Source: CAD feature listing. Evaluate the final solid. Frame: model axes, mm. Face numbers are marked on the shaded views. A direction names the side the tool comes from. Give positions to 0.01 mm unless a question says otherwise; leave off trailing zeros. Loops run counter-clockwise (first coordinate to the right, second up) from the corner with the lowest first, then second, coordinate; pieces in that order, holes last.
from build123d import *

# Parameters (mm, degrees)
F0_R     = 11.176
F0_R_2   = 6.35
F1_DEPTH = 19.05
F2_DEPTH = 6.35
F3_DEPTH = 31.75
F5_DEPTH = 19.05
F6_DEPTH = 50.8


with BuildPart() as f1:
    # F0 (on Top) → F1 (new body)
    with BuildSketch(Plane.XY):
        with BuildLine():
            ThreePointArc((-44.45, 25.4), (-69.85, 0), (-44.45, -25.4))
            Line((-44.45, -25.4), (2.63e-08, -25.4))
            ThreePointArc((2.63e-08, -25.4), (-25.4, -1.24e-08), (1.5e-09, 25.4))
            Line((1.5e-09, 25.4), (-44.45, 25.4))
        make_face()
        with Locations((-44.45, 0)):
            Circle(F0_R, mode=Mode.SUBTRACT)
        with BuildLine():
            ThreePointArc((25.4, 0), (17.9605122514, -17.9605122328), (2.63e-08, -25.4))
            Line((2.63e-08, -25.4), (44.45, -25.4))
            ThreePointArc((44.45, -25.4), (69.85, 0), (44.45, 25.4))
            Line((44.45, 25.4), (1.5e-09, 25.4))
            ThreePointArc((1.5e-09, 25.4), (17.9605122427, 17.9605122416), (25.4, 0))
        make_face()
        with Locations((44.45, 0)):
            Circle(F0_R, mode=Mode.SUBTRACT)
        with Locations((-44.45, 0)):
            Circle(F0_R)
        with Locations((-44.45, 0)):
            Circle(F0_R_2, mode=Mode.SUBTRACT)
        with Locations((44.45, 0)):
            Circle(F0_R)
        with Locations((44.45, 0)):
            Circle(F0_R_2, mode=Mode.SUBTRACT)
        with BuildLine():
            ThreePointArc((1.5e-09, 25.4), (-25.4, -1.24e-08), (2.63e-08, -25.4))
            ThreePointArc((2.63e-08, -25.4), (17.9605122514, -17.9605122328), (25.4, 0))
            ThreePointArc((25.4, 0), (17.9605122427, 17.9605122416), (1.5e-09, 25.4))
        make_face()
    extrude(amount=-F1_DEPTH)

    # F0 (on Top) → F2 (cut)
    with BuildSketch(Plane.XY):
        with Locations((-44.45, 0)):
            Circle(F0_R)
        with Locations((-44.45, 0)):
            Circle(F0_R_2, mode=Mode.SUBTRACT)
        with Locations((44.45, 0)):
            Circle(F0_R)
        with Locations((44.45, 0)):
            Circle(F0_R_2, mode=Mode.SUBTRACT)
    extrude(amount=-F2_DEPTH, mode=Mode.SUBTRACT)

    # F0 (on Top) → F3 (join)
    with BuildSketch(Plane.XY):
        with BuildLine():
            ThreePointArc((1.5e-09, 25.4), (-25.4, -1.24e-08), (2.63e-08, -25.4))
            ThreePointArc((2.63e-08, -25.4), (17.9605122514, -17.9605122328), (25.4, 0))
            ThreePointArc((25.4, 0), (17.9605122427, 17.9605122416), (1.5e-09, 25.4))
        make_face()
    extrude(amount=F3_DEPTH)

    # F4 (on face) → F5 (cut)
    with BuildSketch(Plane.XY.offset(31.75)):
        with BuildLine():
            Line((6.35, -24.5934442484), (6.35, -12.8696814646))
            ThreePointArc((6.35, -12.8696814646), (0, -14.351), (-6.35, -12.8696814646))
            Line((-6.35, -12.8696814646), (-6.35, -24.5934442484))
            ThreePointArc((-6.35, -24.5934442484), (0, -25.4), (6.35, -24.5934442484))
        make_face()
        with BuildLine():
            ThreePointArc((-12.8696814646, -6.35), (-14.351, 0), (-12.8696814646, 6.35))
            Line((-12.8696814646, 6.35), (-24.5934442484, 6.35))
            ThreePointArc((-24.5934442484, 6.35), (-25.4, 0), (-24.5934442484, -6.35))
            Line((-24.5934442484, -6.35), (-12.8696814646, -6.35))
        make_face()
        with BuildLine():
            ThreePointArc((-6.35, 12.8696814646), (0, 14.351), (6.35, 12.8696814646))
            Line((6.35, 12.8696814646), (6.35, 24.5934442484))
            ThreePointArc((6.35, 24.5934442484), (0, 25.4), (-6.35, 24.5934442484))
            Line((-6.35, 24.5934442484), (-6.35, 12.8696814646))
        make_face()
        with BuildLine():
            ThreePointArc((12.8696814646, 6.35), (13.9757647322, 3.260245566), (14.351, 0))
            ThreePointArc((14.351, 0), (13.9757647322, -3.260245566), (12.8696814646, -6.35))
            Line((12.8696814646, -6.35), (24.5934442484, -6.35))
            ThreePointArc((24.5934442484, -6.35), (25.1975542852, -3.2005090291), (25.4, 0))
            ThreePointArc((25.4, 0), (25.1975542852, 3.2005090291), (24.5934442484, 6.35))
            Line((24.5934442484, 6.35), (12.8696814646, 6.35))
        make_face()
    extrude(amount=-F5_DEPTH, mode=Mode.SUBTRACT)

    # F4 (on face) → F6 (cut, through all)
    with BuildSketch(Plane.XY.offset(31.75)):
        with BuildLine():
            ThreePointArc((12.8696814646, -6.35), (13.9757647322, -3.260245566), (14.351, 0))
            ThreePointArc((14.351, 0), (13.9757647322, 3.260245566), (12.8696814646, 6.35))
            ThreePointArc((12.8696814646, 6.35), (10.1476894168, 10.1476894168), (6.35, 12.8696814646))
            ThreePointArc((6.35, 12.8696814646), (0, 14.351), (-6.35, 12.8696814646))
            ThreePointArc((-6.35, 12.8696814646), (-10.1476894168, 10.1476894168), (-12.8696814646, 6.35))
            ThreePointArc((-12.8696814646, 6.35), (-14.351, 0), (-12.8696814646, -6.35))
            ThreePointArc((-12.8696814646, -6.35), (-10.1476894168, -10.1476894168), (-6.35, -12.8696814646))
            ThreePointArc((-6.35, -12.8696814646), (0, -14.351), (6.35, -12.8696814646))
            ThreePointArc((6.35, -12.8696814646), (10.1476894168, -10.1476894168), (12.8696814646, -6.35))
        make_face()
    extrude(amount=-F6_DEPTH, mode=Mode.SUBTRACT)


solid = f1.part
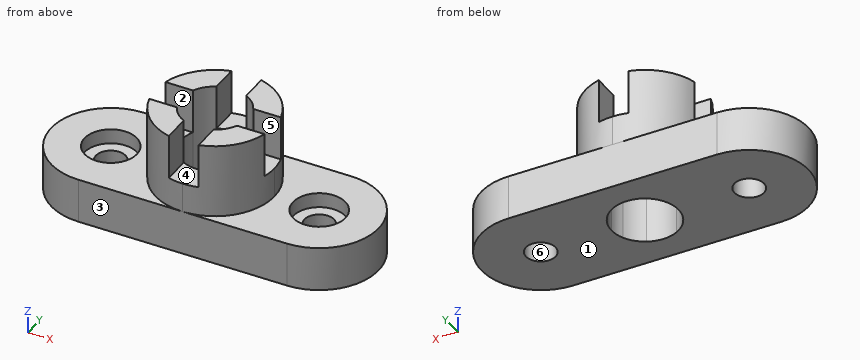
1) Pull-direction query (Y, two-part tool) for the marked faces 1, 2 and 3; classes: released by +Y, released by -Y, zero draft, split by the parting line, or undercut.
Checks:
face 1: zero draft
face 2: undercut
face 3: released by -Y
2) Ray query, probe 1 along Y at (x, z) = (44.45, -15.5); probe 2 along Y at (x, z) = (-44.45, -4.5); probe 3 along Z at (x, y) = (-35, -9). Return the intervals inside material, ascending.
Checks:
probe 1: y = -25.4 to -6.35, 6.35 to 25.4
probe 2: y = -25.4 to -11.18, 11.18 to 25.4
probe 3: z = -19.05 to 0
3) Reachability of the marked faces 4, 5 and 6 from +Z, -Z, +X, -X, +Y, -Y: full face, straight path, thin tool, end or side. Return the list, or none.
Checks:
face 4: +Z, +Y, -Y
face 5: +Z, +X, -X
face 6: +Z, -Z
4) Contact query for flat-ended pins moving along their axis: P1, Ø9.5, axis at y = -18, z = 18, coming from the -X side; P2, Ø3.5, axis at x = -20, z = 19, coming from the -Y side; P3, Ø2, axis at y = 6, z = 21, coming from the -X side; P4, Ø11.5, axis at x = 44.45, y = 0, coming from the -Z side. Output: stop coordinate, or through.
Checks:
P1: stops at x = -21.67
P2: stops at y = -17.67
P3: stops at x = -24.59
P4: passes through
5) Cut plane A-A (z = -4.5). Return loops of the section in (x, y), and give its area (3 significant figures).
Checks:
outline: (-44.45, -25.4) - (44.45, -25.4) arc R25.4 ccw to (44.45, 25.4) - (-44.45, 25.4) arc R25.4 ccw to start; hole circle Ø22.35 at (-44.45, 0); hole circle Ø28.7 at (0, 0); hole circle Ø22.35 at (44.45, 0)
area: 5,110 mm2
6) Cut plane C-C (x = 49). Return loops of the section in (y, z).
Checks:
outline: (-24.99, -19.05) - (-4.43, -19.05) - (-4.43, -6.35) - (-10.21, -6.35) - (-10.21, 0) - (-24.99, 0) - close; (4.43, -19.05) - (24.99, -19.05) - (24.99, 0) - (10.21, 0) - (10.21, -6.35) - (4.43, -6.35) - close
7) Cut plane B-B (z = 11). Return loops of the section in (x, y), and give its area (3 significant figures).
Checks:
outline: circle Ø50.8 at (0, 0); hole circle Ø28.7 at (0, 0)
area: 1,380 mm2
8) Cut plane D-D (y = 4). Return loops of the section in (x, z), and give its area (3 significant figures).
Checks:
outline: (-69.53, -19.05) - (-49.38, -19.05) - (-49.38, -6.35) - (-54.89, -6.35) - (-54.89, 0) - (-69.53, 0) - close; (-39.52, -19.05) - (-13.78, -19.05) - (-13.78, 12.7) - (-25.08, 12.7) - (-25.08, 0) - (-34.01, 0) - (-34.01, -6.35) - (-39.52, -6.35) - close; (13.78, -19.05) - (39.52, -19.05) - (39.52, -6.35) - (34.01, -6.35) - (34.01, 0) - (25.08, 0) - (25.08, 12.7) - (13.78, 12.7) - close; (49.38, -19.05) - (69.53, -19.05) - (69.53, 0) - (54.89, 0) - (54.89, -6.35) - (49.38, -6.35) - close
area: 1,900 mm2
